```python
from build123d import *

# Parameters (mm, degrees)
F0_R     = 35.2243618103
F1_DEPTH = 75.946
F2_R     = 15.3302561211
F3_T     = -2.54


# Not quite as in the source:
# - a shell that OpenCascade refuses in one call is made with other operations: the cavity is built on its own and cut out


with BuildPart() as f1:
    # F0 (on Top) → F1 (new body)
    with BuildSketch(Plane.XY):
        with Locations((-4.9064448103, -47.139827162)):
            Circle(F0_R)
    extrude(amount=F1_DEPTH)

    # F2
    f2_edges = [f1.edges().sort_by_distance(p)[0] for p in [
        (-40.130807, -47.139827, 75.946),
    ]]
    fillet(f2_edges, radius=F2_R)

    # F3: a shell. OpenCascade refuses it in one call, so the cavity is built on its own and cut out:
    # the body offset inwards by the wall thickness, plus a prism from it out through each open face.
    f3_core = offset(f1.part, amount=F3_T, mode=Mode.PRIVATE)
    f3_exits = [f3_core.faces().sort_by_distance(p)[0] for p in [
        (-4.906445, -47.139827, 73.406),
    ]]
    add(f3_core, mode=Mode.SUBTRACT)
    extrude(f3_exits, amount=-F3_T, mode=Mode.SUBTRACT)


solid = f1.part
```
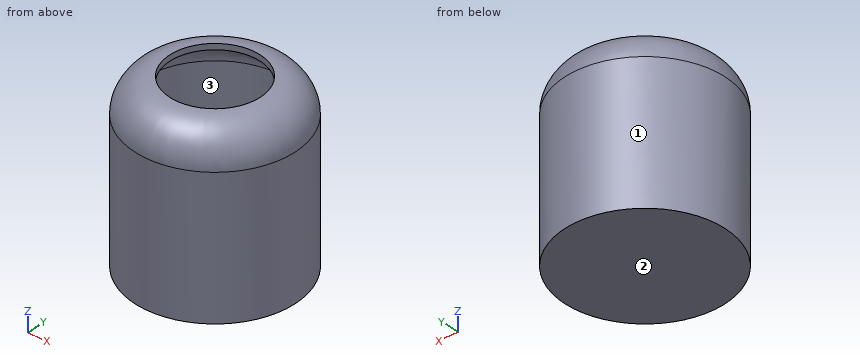
Geometry check sheet. Reference: the model listing, model coordinates, mm. Face numbers are marked on the shaded views. Coordinates: 2 decimals unless noted, no trailing zeros. Order: outer loops, then holes, each group sorted by start corner. A loop starts at its lowest first (then second) coordinate and runs counter-clockwise, first axis right, second up. Notation, with made-up numbers: M 26.25,54 L 67.25,54 A20 ccw 67.25,81 Z; hole C 56,76 d7. An arc over 180 degrees is marked long. Answer as a JSON object with one key per item and string values.
Q1. Cross-section at A-A on z = 20. Record the cut outline in (x, y), and give its area (3 significant figures).
Results are:
{"outline": "C -4.91,-47.14 d70.45; hole C -4.91,-47.14 d65.37", "area": "542 mm²"}
Q2. Depth check by flat-ended pin: pin 1 Ø1.5 at (y, z) = (-44.5, 39) entering from +X; pin 2 Ø1 at (y, z) = (-46, 15) entering from -X (3 decimals); pin 3 Ø5 at (x, y) = (-19.5, -35.5) entering from +Z; pin 4 Ø2 at (x, z) = (3, 52.5) entering from -Y. Enter the tip coordinate at first touch or a pass-through.
Results are:
{"pin 1": "stops at x = 30.27", "pin 2": "stops at x = -40.125", "pin 3": "stops at z = 75.95", "pin 4": "stops at y = -81.68"}
Q3. Release check for a two-part mould opening along X. For the marked faces 1, 2 and 3 record: released by +X, released by -X, zero draft, split by the parting line, or undercut.
Results are:
{"face 1": "split by the parting line", "face 2": "zero draft", "face 3": "undercut"}
Q4. Scan lines: line 1 (Z direction, x = 2.5, y = -28); line 2 (X direction, y = -39.5, z = 34.5); line 3 (Y direction, x = 22.5, z = 63). Record each from-to range of solid material in increasing order.
Results are:
{"line 1": "z = 0 to 2.54, 73.39 to 75.93", "line 2": "x = -39.29 to -36.69, 26.87 to 29.48", "line 3": "y = -68.97 to -64.53, -29.75 to -25.31"}
